Answer from the drawing. Dimensions are ordinates in mm from the lowest x, y and z of the part. A direction names the side the tool comes from. Round coordinates to 2 decimals unless told otherwise and drop trailing zeros. Write each loop counter-clockwise with the first axis right and the second up, starting at its lowest first coordinate (ties: lowest second). Pieces come first, ordered by that corner, then holes. Notation, with made-up numbers: (85.5, 39.25) -> (130.5, 39.25) arc R23 cw to (130.5, 53.25) -> close; hole circle Ø11 at (27, -39.5). An arc over 180 degrees is marked (long way). Return JSON: item names as keys, results as strings. Group by question number.
(1) For the marked faces 1, 2 and 3, determine the directions among +Z, -Z, +X, -X, +Y, -Y from which every point of the face is accessible in a straight line to the end or side of a thin tool.
(2) A cutting plane is placed at C-C on x = 18.5. Give the vertices of the cut face in (y, z).
(3) A cutting plane is placed at A-A on y = 12.5. Give the vertices of the cut face in (x, z), then the cut area to 3 significant figures.
(4) Given pin 1 (1.6 mm diameter, centred on x = 28, z = 1, fed in from +Y); pin 2 (5 mm diameter, centred on x = 13.5, z = 8.5, fed in from +Y); pin 3 (3 mm diameter, centred on y = 10, z = 3, fed in from +X), each flat-ended and moving along its own axis, determine where each tip first touches the part or whether it passes through.
(5) The mould has two halves that part along Y. Classify the marked faces 4, 5 and 6: released by +Y, released by -Y, zero draft, split by the parting line, or undercut.
(6) A cutting plane is placed at D-D on y = 6.25. Give the vertices of the cut face in (x, z), then the cut area to 3 significant figures.
(7) Straight lines are drawn through the part: line 1 (Z direction, x = 19.25, y = 9.5); line 2 (Y direction, x = 6, z = 8.25). For each, find the intervals that lie inside material, in ascending order.
(8) A cutting plane is placed at B-B on z = 7.75. Give the vertices of the cut face in (x, y).
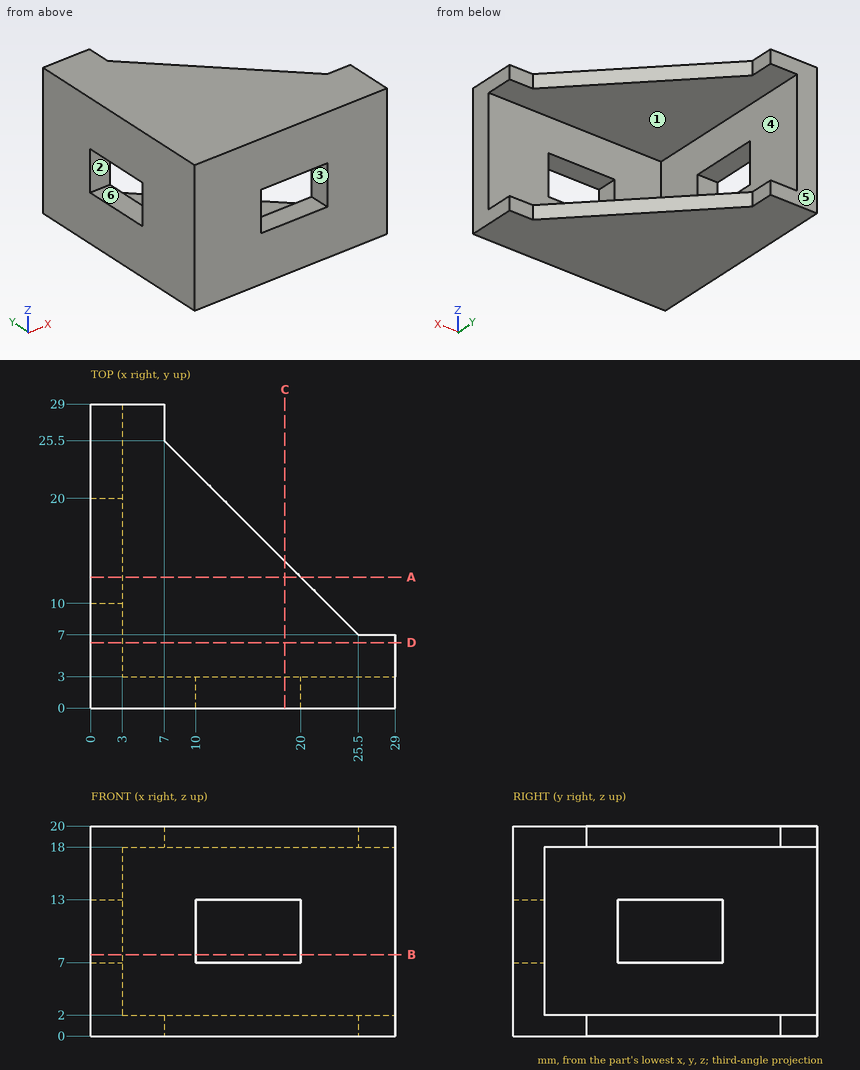
Checks:
{
 "1": {"face 1": "+X, +Y", "face 2": "+X, -X", "face 3": "+Y, -Y"},
 "2": {"outline": "(0, 0) -> (14, 0) -> (14, 2) -> (3, 2) -> (3, 7) -> (0, 7) -> close; (0, 13) -> (3, 13) -> (3, 18) -> (14, 18) -> (14, 20) -> (0, 20) -> close"},
 "3": {"outline": "(0, 0) -> (20, 0) -> (20, 2) -> (3, 2) -> (3, 7) -> (0, 7) -> close; (0, 13) -> (3, 13) -> (3, 18) -> (20, 18) -> (20, 20) -> (0, 20) -> close", "area": "110 mm^2"},
 "4": {"pin 1": "stops at y = 7", "pin 2": "stops at y = 3", "pin 3": "stops at x = 23.62"},
 "5": {"face 4": "zero draft", "face 5": "released by +Y", "face 6": "undercut"},
 "6": {"outline": "(0, 0) -> (29, 0) -> (29, 2) -> (3, 2) -> (3, 18) -> (29, 18) -> (29, 20) -> (0, 20) -> close", "area": "164 mm^2"},
 "7": {"line 1": "z = 0 to 2, 18 to 20", "line 2": "y = 0 to 3"},
 "8": {"outline": "(0, 0) -> (10, 0) -> (10, 3) -> (3, 3) -> (3, 10) -> (0, 10) -> close; (0, 20) -> (3, 20) -> (3, 29) -> (0, 29) -> close; (20, 0) -> (29, 0) -> (29, 3) -> (20, 3) -> close"}
}
